The model under review builds one solid part; all positions refer to its coordinate system, in mm. Round coordinates to 2 decimals unless told otherwise and drop trailing zeros. Write each loop counter-clockwise with the first axis right and the second up, starting at its lowest first coordinate (ties: lowest second). Pieces come first, ordered by that corner, then holes. Notation, with made-up numbers: (4, 11) -> (44, 11) arc R34 ccw to (44, 48) -> close; hole circle Ø11 at (56, -10). An arc over 180 degrees is marked (long way). Answer in a Markdown table with one row per item. Add a question column.
```python
from build123d import *

# Parameters (mm, degrees)
BOSS_EXTRUDE1_START = -4
BOSS_EXTRUDE1_DEPTH = 4
CIRPATTERN2_COUNT   = 2
CIRPATTERN2_ANGLE   = 55
CUT_EXTRUDE1_DEPTH  = 9
FILLET1_R           = 14


with BuildPart() as part:
    # Sketch1 → Revolve1 (revolve)
    with BuildSketch(Plane.XY, mode=Mode.PRIVATE) as revolve1_sk:
        with BuildLine():
            Line((111, 12), (139, 12))
            Line((139, 12), (139, 0))
            Line((139, 0), (132.937253933, 0))
            ThreePointArc((132.937253933, 0), (125, 7), (117.062746067, 0))
            Line((117.062746067, 0), (111, 0))
            Line((111, 0), (111, 12))
        make_face()
    revolve(revolve1_sk.sketch.rotate(Axis((0, 4.511025306, 0), (0, 1, 0)), 90), axis=Axis((0, 4.511025306, 0), (0, 1, 0)))

    # Sketch2 → Boss-Extrude1 (add)
    with BuildSketch(Plane.XZ.offset(BOSS_EXTRUDE1_START)):
        with BuildLine():
            Line((82.734356473, 57.931220071), (90.925876916, 63.666984435))
            ThreePointArc((90.925876916, 63.666984435), (93.616450485, 59.640256526), (96.12881982, 55.5))
            Line((96.12881982, 55.5), (87.468565782, 50.5))
            ThreePointArc((87.468565782, 50.5), (85.182536027, 54.267260443), (82.734356473, 57.931220071))
        make_face()
    boss_extrude1 = extrude(amount=BOSS_EXTRUDE1_DEPTH)

    # CirPattern2: Boss-Extrude1 ×2 about axis
    cirpattern2_axis = Axis((0, 0, 0), (0, -1, 0))
    for i in range(1, CIRPATTERN2_COUNT):
        add(boss_extrude1.rotate(cirpattern2_axis, i * CIRPATTERN2_ANGLE / (CIRPATTERN2_COUNT - 1)))

    # Sketch5 → Cut-Extrude1 (cut)
    with BuildSketch(Plane.XZ):
        Polygon((-75.247171131, 81.601858047), (-79.64873019, 83.973835671), (-78.937136903, 85.294303389), (-74.070295271, 82.671587371), (-71.895448203, 81.499573429), (-72.60704149, 80.179105712), align=None)
    extrude(amount=-CUT_EXTRUDE1_DEPTH, mode=Mode.SUBTRACT)

    # Fillet1
    # the kernel refuses this fillet: 14 mm, written as the material it takes off along each edge
    with BuildSketch(Plane(origin=(0, 4, 0), x_dir=(0.9607578733888479, 0, 0.2773883716404464), z_dir=(0.2773883716404464, 0, -0.9607578733888479))) as fillet1_piece_1:
        with BuildLine():
            CenterArc((110.797958971, 14), FILLET1_R, 225.584691403, 44.415308597)
            Line((110.797958971, 0), (110.797958971, -0.28))
            Line((110.797958971, -0.28), (101, -0.28))
            Line((101, -0.28), (100.72, 0))
            ThreePointArc((100.72, 0), (100.72, 2), (100.804040821, 3.8))
            Line((100.804040821, 3.8), (101, 4))
        make_face()
    revolve(axis=Axis((0, 4, 0), (0, -1, 0)), revolution_arc=32.79120756, mode=Mode.SUBTRACT)
    with BuildSketch(Plane(origin=(0, 4, 0), x_dir=(0.32384482552331617, 0, 0.9461102097439669), z_dir=(0.9461102097439669, 0, -0.32384482552331617))) as fillet1_piece_2:
        with BuildLine():
            CenterArc((110.797958971, 14), FILLET1_R, 225.584691403, 44.415308597)
            Line((110.797958971, 0), (110.797958971, -0.28))
            Line((110.797958971, -0.28), (101, -0.28))
            Line((101, -0.28), (100.72, 0))
            ThreePointArc((100.72, 0), (100.72, 2), (100.804040821, 3.8))
            Line((100.804040821, 3.8), (101, 4))
        make_face()
    revolve(axis=Axis((0, 4, 0), (0, -1, 0)), revolution_arc=32.79120756, mode=Mode.SUBTRACT)


solid = part.part
```
1. Insertion check: pin 1 Ø4 at (y, z) = (1.5, 108) entering from +X; pin 2 Ø4 at (x, y) = (81.5, 5.5) entering from -Z; pin 3 Ø1.2 at (y, z) = (1, 104) entering from -X. Each pin has a flat end and moves straight along its axis. Give the tip position at first contact, or say it passes through.
2. Mouldability with a two-part tool opening along X and no side actions: class faces 1 (the cylindrical face through (98.476, 6.084, -51.22)), 2 (the cylindrical face through (-41.75, 5.92, -132.58)), 3 (the flat face through (61, 12, -93)) as pulls with the +X half, pulls with the -X half, needs draft (parallel to the pull), parting line crosses it, or undercut.
3. For L1, parallel to X at y = 9.25, z = 0; L2, parallel to X at y = 5.75, z = -79.5; L3, parallel to Z at x = 53, y = 2.5, list the stretches that pass through material, from the lowest coordinate up.
4. Add section A-A on z = 0. Write out the cut boundary in (x, y), plus the area to 3 significant figures.
Filled in:
| question | item | result |
|---|---|---|
| 1 | pin 1 | x = 89.92 |
| 1 | pin 2 | z = -114.02 |
| 1 | pin 3 | x = -92.89 |
| 2 | face 1 | undercut |
| 2 | face 2 | parting line crosses it |
| 2 | face 3 | needs draft |
| 3 | L1 | -139 to -111, 111 to 139 |
| 3 | L2 | -114.02 to -101.96, -90.83 to -77.46, 77.46 to 90.83, 101.96 to 114.02 |
| 3 | L3 | -128.5 to -121.1, -105.21 to -97.53, 97.53 to 105.21, 121.1 to 128.5 |
| 4 | outline | (-139, 0) -> (-132.94, 0) arc R8 cw to (-117.06, 0) -> (-111, 0) -> (-111, 12) -> (-139, 12) -> close; (111, 0) -> (117.06, 0) arc R8 cw to (132.94, 0) -> (139, 0) -> (139, 12) -> (111, 12) -> close |
| 4 | area | 503 mm² |
